Can you work these out from the model? Positions are in its coordinate system, mm. A direction names the side the tool comes from. Round coordinates to 2 decimals unless told otherwise and drop trailing zeros. Write each loop counter-clockwise with the first axis right and the second up, starting at its lowest first coordinate (ties: lowest second). Pieces come first, ordered by that corner, then holes. Notation, with made-up numbers: (-31.5, 83.25) -> (5.5, 83.25) arc R11 ccw to (5.5, 103.25) -> close; hole circle Ø7 at (1, -23.75). An arc over 180 degrees is marked (long way). Use CSV: the item, a comma, the result in double quotes.
```python
from build123d import *

# Parameters (mm, degrees)
BOX_W        = 35
BOX_H        = 14.5
BOX_DEPTH    = 3
SKETCH006_W  = 1.8
SKETCH006_H  = 10
PAD002_DEPTH = 12
SKETCH007_W  = 2
SKETCH007_H  = 10
PAD003_DEPTH = 12


with BuildPart() as part:
    # Box → Box (new body)
    with BuildSketch(Plane(origin=(0, -8.5, 10), x_dir=(1, 0, 0), z_dir=(0, 0, 1))):
        with Locations((17.5, 7.25)):
            Rectangle(BOX_W, BOX_H)
    extrude(amount=BOX_DEPTH)

    # Sketch006 → Pad002 (new body)
    with BuildSketch(Plane(origin=(0, -8.5, 10), x_dir=(0, -1, 0), z_dir=(-1, 0, 0))):
        with Locations((-13.6, -5)):
            Rectangle(SKETCH006_W, SKETCH006_H)
        with Locations((-0.9, -5)):
            Rectangle(SKETCH006_W, SKETCH006_H)
    extrude(amount=-PAD002_DEPTH)

    # Sketch007 → Pad003 (new body)
    with BuildSketch(Plane(origin=(35, -8.5, 10), x_dir=(0, 1, 0), z_dir=(1, 0, 0))):
        with Locations((13.5, -5)):
            Rectangle(SKETCH007_W, SKETCH007_H)
        with Locations((1, -5)):
            Rectangle(SKETCH007_W, SKETCH007_H)
    extrude(amount=-PAD003_DEPTH)


solid = part.part
```
Q1. Suppose I cut it at D-D (y = -2.25). Write out the boundary of the cut face in (x, z).
Resolved:
outline,"(0, 10) -> (35, 10) -> (35, 13) -> (0, 13) -> close"
Q2. Suppose I cut it at A-A (z = 6.75). Write out the boundary of the cut face in (x, y), and give its area (3 significant figures).
Resolved:
outline,"(0, -8.5) -> (12, -8.5) -> (12, -6.7) -> (0, -6.7) -> close; (0, 4.2) -> (12, 4.2) -> (12, 6) -> (0, 6) -> close; (23, -8.5) -> (35, -8.5) -> (35, -6.5) -> (23, -6.5) -> close; (23, 4) -> (35, 4) -> (35, 6) -> (23, 6) -> close"
area,"91.2 mm^2"
Q3. On a 3-axis mill with a long thin cutter (end or side, diameter ignored), from which of +Z, -Z, +X, -X, +Y, -Y can I reach the whole of each face in a straight line? I mean faces 1 (the face through (29, 4, 5)), 2 (the face through (6, 4.2, 5)), 3 (the face through (12, 5, 5)). Say none if no direction works.
Resolved:
face 1,"-Z, +X, -X"
face 2,"-Z, -X"
face 3,"-Z, +Y, -Y"
Q4. If we mould it in two halves opening along X, with no side actions, what happens to faces 4 (the face through (35, -1, 11)), 5 (the face through (17, -8.5, 11)), 6 (the face through (23, -8, 5))? For each: released by +X, released by -X, zero draft, split by the parting line, or undercut.
Resolved:
face 4,"released by +X"
face 5,"zero draft"
face 6,"undercut"
Q5. Suppose I cut it at B-B (x = 10.5). Write out the boundary of the cut face in (y, z), and give its area (3 significant figures).
Resolved:
outline,"(-8.5, 0) -> (-6.7, 0) -> (-6.7, 10) -> (4.2, 10) -> (4.2, 0) -> (6, 0) -> (6, 13) -> (-8.5, 13) -> close"
area,"79.5 mm^2"
Q6. Suppose I cut it at C-C (y = 4.75). Write out the boundary of the cut face in (x, z).
Resolved:
outline,"(0, 0) -> (12, 0) -> (12, 10) -> (23, 10) -> (23, 0) -> (35, 0) -> (35, 13) -> (0, 13) -> close"
Q7. Please list where these lines run through material, in increasing order: probe 1 along Y at (x, z) = (8.5, 6.25); probe 2 along Y at (x, z) = (30.5, 6.75); probe 3 along Z at (x, y) = (26.5, 1.5).
Resolved:
probe 1,"y = -8.5 to -6.7, 4.2 to 6"
probe 2,"y = -8.5 to -6.5, 4 to 6"
probe 3,"z = 10 to 13"
